Geometry: see drawing. Coordinates: mm, zero at the bounding-box minimum. Coordinates: 2 decimals unless noted, no trailing zeros. Order: outer loops, then holes, each group sorted by start corner. A loop starts at its lowest first (then second) coordinate and runs counter-clockwise, first axis right, second up.
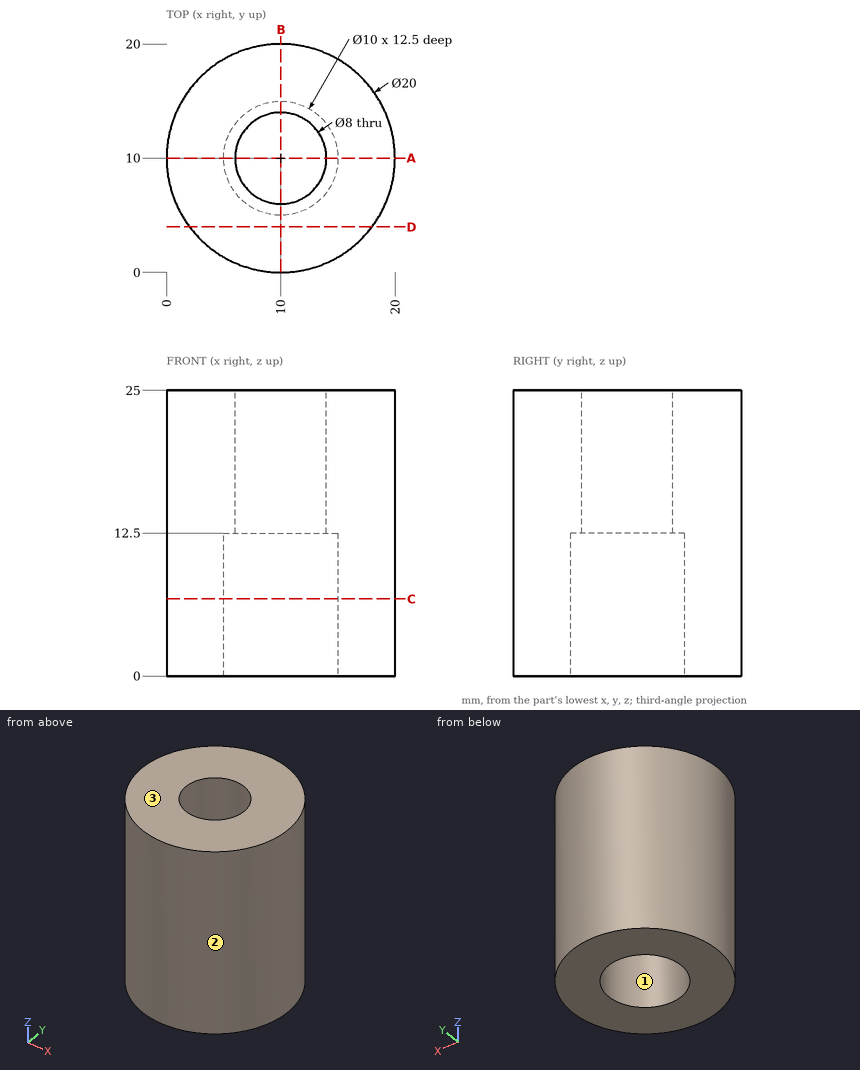
Q1. Material intervals for line 1 along Y through (x, z) = (10, 8.75); line 2 along Y through (x, z) = (10, 21.5); line 3 along Z through (x, y) = (8.75, 5.75), sorted ascending.
Solutions:
line 1: y = 0 to 5, 15 to 20
line 2: y = 0 to 6, 14 to 20
line 3: z = 12.5 to 25
Q2. Pull-direction query (Y, two-part tool) for the marked faces 1, 2 and 3; classes: pulls with the +Y half, pulls with the -Y half, needs draft (parallel to the pull), parting line crosses it, or undercut.
Solutions:
face 1: undercut
face 2: parting line crosses it
face 3: needs draft
Q3. Section query A-A on y = 10. Output: boundary loops of the cut face in (x, z), plus the area to 3 significant figures.
Solutions:
outline: (0, 0) - (5, 0) - (5, 12.5) - (6, 12.5) - (6, 25) - (0, 25) - close; (14, 12.5) - (15, 12.5) - (15, 0) - (20, 0) - (20, 25) - (14, 25) - close
area: 275 mm2
Q4. Section query C-C on z = 6.75. Output: boundary loops of the cut face in (x, y).
Solutions:
outline: circle Ø20 at (10, 10); hole circle Ø10 at (10, 10)
Q5. Pin query (flat end, axial travel): P1, Ø8, axis at y = 18, z = 18, coming from the -X side; P2, Ø5, axis at x = 11, y = 11.5, coming from the -Z side; P3, Ø2, axis at x = 13, z = 19, coming from the +Y side. Return the tip coordinate at first contact, or that it passes through.
Solutions:
P1: stops at x = 0.83
P2: stops at z = 12.5
P3: stops at y = 19.8
Q6. Section query D-D on y = 4. Output: boundary loops of the cut face in (x, z).
Solutions:
outline: (2, 0) - (18, 0) - (18, 25) - (2, 25) - close
